from build123d import *

# Parameters (mm, degrees)
BOSS_EXTRUDE1_DEPTH = 4
SKETCH2_R           = 1.5
BOSS_EXTRUDE2_DEPTH = 4.2
SKETCH3_R           = 1.5
BOSS_EXTRUDE3_DEPTH = 10.7


with BuildPart() as part:
    # Sketch1 → Boss-Extrude1 (new body)
    with BuildSketch(Plane(origin=(0, 0, 0), x_dir=(0, 0, -1), z_dir=(1, 0, 0))):
        with BuildLine():
            ThreePointArc((-0.761904762, 1.849189318), (-1.849189318, -0.761904762), (0.761904762, -1.849189318))
            ThreePointArc((0.761904762, -1.849189318), (16, 1.167024322), (31.238095238, -1.849189318))
            ThreePointArc((31.238095238, -1.849189318), (33.849189318, -0.761904762), (32.761904762, 1.849189318))
            ThreePointArc((32.761904762, 1.849189318), (16, 5.167024322), (-0.761904762, 1.849189318))
        make_face()
    extrude(amount=BOSS_EXTRUDE1_DEPTH)

    # Sketch2 → Boss-Extrude2 (add)
    with BuildSketch(Plane(origin=(4, 0, 0), x_dir=(0, 0, -1), z_dir=(1, 0, 0))):
        with Locations(Location((32, 0, 0), (0, 0, 180))):
            Circle(SKETCH2_R)
    extrude(amount=BOSS_EXTRUDE2_DEPTH)

    # Sketch3 → Boss-Extrude3 (add)
    with BuildSketch(Plane.ZY):
        Circle(SKETCH3_R)
    extrude(amount=BOSS_EXTRUDE3_DEPTH)


solid = part.part
Verification items for the finished model (mm, model axes). A direction names the side the tool comes from. Coordinates: 2 decimals unless noted, no trailing zeros. Order: outer loops, then holes, each group sorted by start corner. A loop starts at its lowest first (then second) coordinate and runs counter-clockwise, first axis right, second up. Notation, with made-up numbers: M 71,-11 L 110,-11 A30 cw 110,13 Z; hole C 29,7 d9. An arc over 180 degrees is marked long. One line per item, written item: value. Start each with the question number.
Item 1: Access from +Z, -Z, +X, -X, +Y, -Y to the whole of each face (thin tool, end or side, straight path). Record for faces 4 (the cylindrical face through (1.972, 5.166, -16.241)), 5 (the cylindrical face through (-5.28, 0.07, -1.5)).
Item 2: Sectioned sample at A-A (y = 0). Enter the section's corners in (x, z).
Item 3: Sectioned sample at C-C (x = 2.25). Enter the section's corners in (y, z), then the cut area to 3 significant figures.
Item 4: Sectioned sample at D-D (y = 2.75). Enter the section's corners in (x, z).
Item 5: Sectioned sample at B-B (z = -32). Enter the section's corners in (x, y), then the cut area to 3 significant figures.
Item 6: Scan lines: probe 1 along Y at (x, z) = (-6.5, 0); probe 2 along X at (y, z) = (3.5, -11); probe 3 along Y at (x, z) = (2.25, -16). Record each from-to range of solid material in increasing order.
Item 7: Mould release check, pull along Z, two halves, no side actions. Record for faces 1 (the cylindrical face through (6.1, 0.9, -33.2)), 2 (the cylindrical face through (1.972, 1.166, -15.781)), 3 (the flat face through (4, 2, -16)): released by +Z, released by -Z, zero draft, split by the parting line, or undercut.
Item 8: Gauge pin test, flat ends, axial feed: pin 1 (3 mm diameter, centred on y = 0, z = -30, fed in from -X); pin 2 (1 mm diameter, centred on y = -1, z = -15, fed in from +X); pin 3 (2 mm diameter, centred on y = 1.5, z = -19, fed in from +X). Record the tip position at first contact, or that the pin passes through.
Conclusion:
1. face 4: +X, -X, +Y
1. face 5: -X
2. outline: M -10.7,-1.5 L 0,-1.5 L 0,-6.41 L 4,-6.41 L 4,2 L 0,2 L 0,1.5 L -10.7,1.5 Z; M 0,-34 L 4,-34 L 4,-33.5 L 8.2,-33.5 L 8.2,-30.5 L 4,-30.5 L 4,-25.59 L 0,-25.59 Z
3. outline: M -1.85,-31.24 A2 ccw 1.85,-32.76 A44 ccw 1.85,0.76 A2 ccw -1.85,-0.76 A40 cw Z
3. area: 144 mm^2
4. outline: M 0,-30.38 L 4,-30.38 L 4,-1.62 L 0,-1.62 Z
5. outline: M 0,-2 L 4,-2 L 4,-1.5 L 8.2,-1.5 L 8.2,1.5 L 4,1.5 L 4,2.15 L 0,2.15 Z
5. area: 29.2 mm^2
6. probe 1: y = -1.5 to 1.5
6. probe 2: x = 0 to 4
6. probe 3: y = 1.17 to 5.17
7. face 1: split by the parting line
7. face 2: undercut
7. face 3: zero draft
8. pin 1: stops at x = 0
8. pin 2: passes through
8. pin 3: stops at x = 4
